from build123d import *

# Parameters (mm, degrees)
SKETCH1_W           = 70
SKETCH1_H           = 60
BOSS_EXTRUDE1_DEPTH = 3
SKETCH2_W           = 15
SKETCH2_H           = 9
CUT_EXTRUDE1_DEPTH  = 3
SKETCH3_W           = 20
SKETCH3_H           = 3
CUT_EXTRUDE2_DEPTH  = 3
SKETCH4_W           = 3
SKETCH4_H           = 20
BOSS_EXTRUDE2_DEPTH = 3


with BuildPart() as part:
    # Sketch1 → Boss-Extrude1 (new body)
    with BuildSketch(Plane.XY):
        Rectangle(SKETCH1_W, SKETCH1_H)
    extrude(amount=BOSS_EXTRUDE1_DEPTH)

    # Sketch2 → Cut-Extrude1 (cut)
    with BuildSketch(Plane.XY.offset(3)):
        with Locations((4, 9.7)):
            Rectangle(SKETCH2_W, SKETCH2_H)
    extrude(amount=-CUT_EXTRUDE1_DEPTH, mode=Mode.SUBTRACT)

    # Sketch3 → Cut-Extrude2 (cut)
    with BuildSketch(Plane.XY.offset(3)):
        with Locations((0, 2.5)):
            Rectangle(SKETCH3_W, SKETCH3_H)
    extrude(amount=-CUT_EXTRUDE2_DEPTH, mode=Mode.SUBTRACT)

    # Sketch4 → Boss-Extrude2 (add)
    with BuildSketch(Plane.XY.offset(3)):
        with Locations((36.5, 0)):
            Rectangle(SKETCH4_W, SKETCH4_H)
        with Locations((-36.5, 0)):
            Rectangle(SKETCH4_W, SKETCH4_H)
    extrude(amount=-BOSS_EXTRUDE2_DEPTH)


solid = part.part
Could you check a few things on this model? Use its own coordinates, in mm. A direction names the side the tool comes from. Coordinates: 2 decimals unless noted, no trailing zeros. Order: outer loops, then holes, each group sorted by start corner. A loop starts at its lowest first (then second) coordinate and runs counter-clockwise, first axis right, second up. Notation, with made-up numbers: (-4.75, 56) -> (45.25, 56) arc R11 ccw to (45.25, 75) -> close; hole circle Ø7 at (54.5, -4). An arc over 180 degrees is marked (long way). One line per question, with ' | ' between items.
Q1. Thinking about a two-plate mould opening in X: for faces 5 (the face through (-35, 20, 1)), 6 (the face through (-1, 0, 0)), 7 (the face through (-3.5, 10, 2)), 8 (the face through (35, 20, 1)), which applies, pulls with the +X half, pulls with the -X half, needs draft (parallel to the pull), parting line crosses it, or undercut?
Return value:
face 5: pulls with the -X half | face 6: needs draft | face 7: undercut | face 8: pulls with the +X half
Q2. Imagine slicing it at C-C on y = 2. Please give me the cut outline in (x, z), and give its area (3 significant figures).
Return value:
outline: (-38, 0) -> (-10, 0) -> (-10, 3) -> (-38, 3) -> close; (10, 0) -> (38, 0) -> (38, 3) -> (10, 3) -> close | area: 168 mm²
Q3. Imagine slicing it at B-B on z = 0.65. Please give me the cut outline in (x, y), and give its area (4 significant figures).
Return value:
outline: (-38, -10) -> (-35, -10) -> (-35, -30) -> (35, -30) -> (35, -10) -> (38, -10) -> (38, 10) -> (35, 10) -> (35, 30) -> (-35, 30) -> (-35, 10) -> (-38, 10) -> close; hole (-10, 1) -> (10, 1) -> (10, 4) -> (-10, 4) -> close; hole (-3.5, 5.2) -> (11.5, 5.2) -> (11.5, 14.2) -> (-3.5, 14.2) -> close | area: 4,125 mm²
Q4. Imagine slicing it at A-A on y = 12.5. Please give me the cut outline in (x, z), and give its area (3 significant figures).
Return value:
outline: (-35, 0) -> (-3.5, 0) -> (-3.5, 3) -> (-35, 3) -> close; (11.5, 0) -> (35, 0) -> (35, 3) -> (11.5, 3) -> close | area: 165 mm²
Q5. Imagine slicing it at D-D on y = -26. Please give me the cut outline in (x, z).
Return value:
outline: (-35, 0) -> (35, 0) -> (35, 3) -> (-35, 3) -> close
Q6. On a 3-axis mill with a long thin cutter (end or side, diameter ignored), from which of +Z, -Z, +X, -X, +Y, -Y can I reach the whole of each face in a straight line? I mean faces 1 (the face through (36, -10, 2)), 2 (the face through (4, 5.2, 2)), 3 (the face through (-37, -10, 2)), 4 (the face through (-37, 10, 2)). Say none if no direction works.
Return value:
face 1: +Z, -Z, +X, -Y | face 2: +Z, -Z | face 3: +Z, -Z, -X, -Y | face 4: +Z, -Z, -X, +Y
Q7. I'm going to push flat-ended pins straight in: P1, Ø1.5, axis at y = -21.5, z = 1.5, coming from the -X side; P2, Ø1.5, axis at x = 36, z = 2, coming from the -Y side. Where does each tip first touch, or does it pass through?
Return value:
P1: x = -35 | P2: y = -10
Q8. If I drill on L1, parallel to Y at x = 6, z = 0.2; L2, parallel to X at y = 8, z = 2.4; L3, parallel to Y at x = -5.5, z = 1.6, over which ranges is the centre line in solid material (lowest first)?
Return value:
L1: -30 to 1, 4 to 5.2, 14.2 to 30 | L2: -38 to -3.5, 11.5 to 38 | L3: -30 to 1, 4 to 30
